```python
from build123d import *

# Parameters (mm, degrees)
F2_R = 0.69999
F3_R = 1


# Not quite as in the source:
# - a fillet or chamfer is up to 0.001 mm smaller than in the source, because OpenCascade refuses the exact size


with BuildPart() as f1:
    # F0 (on Front) → F1 (revolve)
    with BuildSketch(Plane.XZ):
        Polygon((0, 9), (0, 8), (4.3, 8), (4.3, 0), (5.7, 0), (5.7, 9), align=None)
    revolve(axis=Axis((0, 0, 8.5), (0, 0, -1)))

    # F2 (radius 0.7 in the source; OpenCascade refuses exactly that, so slightly less here)
    f2_edges = [f1.edges().sort_by_distance(p)[0] for p in [
        (-5.7, 0, 0),
        (-4.3, 0, 0),
        (-5.7, 0, 9),
    ]]
    fillet(f2_edges, radius=F2_R)

    # F3
    f3_edges = [f1.edges().sort_by_distance(p)[0] for p in [
        (-4.3, 0, 8),
    ]]
    fillet(f3_edges, radius=F3_R)


solid = f1.part
```
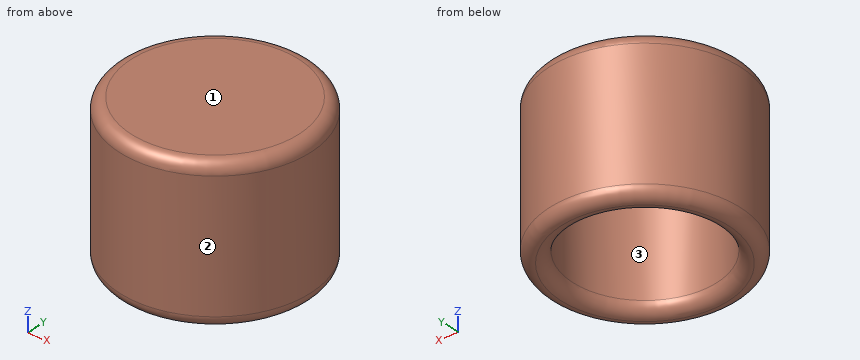
Check sheet for the modelled part. Datum: model origin and axes. Units: mm. Face numbers are marked on the shaded views. Coordinates: 2 decimals unless noted, no trailing zeros. Order: outer loops, then holes, each group sorted by start corner. A loop starts at its lowest first (then second) coordinate and runs counter-clockwise, first axis right, second up. Notation, with made-up numbers: M 29.5,-38 L 82.5,-38 A13 ccw 82.5,-13 Z; hole C 11,58.25 d2. An arc over 180 degrees is marked long. One line per question, with ' | ' between items. Start each with the question number.
Item 1: Sectioned sample at C-C on z = 2. Record the cut outline in (x, y), and give its area (3 significant figures).
Item 2: Gauge pin test, flat ends, axial feed: P1, Ø1, axis at x = 4, y = 1.5, coming from the -Z side; P2, Ø1, axis at x = 4.5, z = 3, coming from the -Y side; P3, Ø2, axis at x = -4.5, z = 8, coming from the +Y side. Record the tip position at first contact, or that the pin passes through.
Item 3: Mould release check, pull along X, two halves, no side actions. Record for the marked faces 1, 2 and 3: pulls with the +X half, pulls with the -X half, needs draft (parallel to the pull), parting line crosses it, or undercut.
Item 4: Sectioned sample at D-D on z = 7.5. Record the cut outline in (x, y), and give its area (3 significant figures).
Item 5: Material ranges on line 1 (Y direction, x = 0, z = 4); line 2 (Z direction, x = 2.25, y = 1.5), recorded low to high.
Answer below:
1) outline: C 0,0 d11.4; hole C 0,0 d8.6 | area: 44.0 mm^2
2) P1: stops at z = 0.04 | P2: stops at y = -4.06 | P3: stops at y = 4.5
3) face 1: needs draft | face 2: parting line crosses it | face 3: undercut
4) outline: C 0,0 d11.4; hole C 0,0 d8.33 | area: 47.5 mm^2
5) line 1: y = -5.7 to -4.3, 4.3 to 5.7 | line 2: z = 8 to 9
